from build123d import *

# Parameters (mm, degrees)
SKETCH2_W                          = 128
SKETCH2_H                          = 80
BASE_PLATE_DEPTH                   = 10
PIVOT_PEDESTAL_START               = 10
SKETCH3_R                          = 6
PIVOT_PEDESTAL_DEPTH               = 16
SKETCH4_R                          = 2.7
PIVOT_CLEARANCE_DEPTH              = 26
SKETCH5_R                          = 3.15
LOCATOR_CLEARANCE_DEPTH            = 10
SKETCH6_R                          = 3.15
CUT_EXTRUDE3_DEPTH                 = 10
SKETCH7_R                          = 3.15
SIDE_LOCATOR_CLEARANCE_DEPTH       = 10
LOCATOR_SHOULDER_COUNTERBORE_START = 8
SKETCH8_R                          = 4.1
LOCATOR_SHOULDER_COUNTERBORE_DEPTH = 2
CUT_EXTRUDE6_START                 = 8
SKETCH9_R                          = 4.1
CUT_EXTRUDE6_DEPTH                 = 2
SIDE_SHOULDER_COUNTERBORE_START    = 8
SKETCH10_R                         = 4.1
SIDE_SHOULDER_COUNTERBORE_DEPTH    = 2
SKETCH11_R                         = 3.3
BENCH_MOUNT_M6_CLEARANCE_DEPTH     = 10
SKETCH12_R                         = 3.3
CUT_EXTRUDE9_DEPTH                 = 10
SKETCH13_R                         = 3.3
CUT_EXTRUDE10_DEPTH                = 10
SKETCH14_R                         = 3.3
CUT_EXTRUDE11_DEPTH                = 10


with BuildPart() as part:
    # Sketch2 → Base_plate (new body)
    with BuildSketch(Plane.XY):
        Rectangle(SKETCH2_W, SKETCH2_H)
    extrude(amount=BASE_PLATE_DEPTH)

    # Sketch3 → Pivot_pedestal (add)
    with BuildSketch(Plane.XY.offset(PIVOT_PEDESTAL_START)):
        with Locations(Location((-35, 0, 0), (0, 0, 180))):
            Circle(SKETCH3_R)
    extrude(amount=PIVOT_PEDESTAL_DEPTH)

    # Sketch4 → Pivot_clearance (cut)
    with BuildSketch(Plane.XY):
        with Locations(Location((-35, 0, 0), (0, 0, 180))):
            Circle(SKETCH4_R)
    extrude(amount=PIVOT_CLEARANCE_DEPTH, mode=Mode.SUBTRACT)

    # Sketch5 → Locator_clearance (cut)
    with BuildSketch(Plane.XY):
        with Locations((-10, 15)):
            Circle(SKETCH5_R)
    extrude(amount=LOCATOR_CLEARANCE_DEPTH, mode=Mode.SUBTRACT)

    # Sketch6 → Cut-Extrude3 (cut)
    with BuildSketch(Plane.XY):
        with Locations((10, 15)):
            Circle(SKETCH6_R)
    extrude(amount=CUT_EXTRUDE3_DEPTH, mode=Mode.SUBTRACT)

    # Sketch7 → Side_locator_clearance (cut)
    with BuildSketch(Plane.XY):
        with Locations((-18, -5)):
            Circle(SKETCH7_R)
    extrude(amount=SIDE_LOCATOR_CLEARANCE_DEPTH, mode=Mode.SUBTRACT)

    # Sketch8 → Locator_shoulder_counterbore (cut)
    with BuildSketch(Plane.XY.offset(LOCATOR_SHOULDER_COUNTERBORE_START)):
        with Locations((-10, 15)):
            Circle(SKETCH8_R)
    extrude(amount=LOCATOR_SHOULDER_COUNTERBORE_DEPTH, mode=Mode.SUBTRACT)

    # Sketch9 → Cut-Extrude6 (cut)
    with BuildSketch(Plane.XY.offset(CUT_EXTRUDE6_START)):
        with Locations((10, 15)):
            Circle(SKETCH9_R)
    extrude(amount=CUT_EXTRUDE6_DEPTH, mode=Mode.SUBTRACT)

    # Sketch10 → Side_shoulder_counterbore (cut)
    with BuildSketch(Plane.XY.offset(SIDE_SHOULDER_COUNTERBORE_START)):
        with Locations((-18, -5)):
            Circle(SKETCH10_R)
    extrude(amount=SIDE_SHOULDER_COUNTERBORE_DEPTH, mode=Mode.SUBTRACT)

    # Sketch11 → Bench_mount_M6_clearance (cut)
    with BuildSketch(Plane.XY):
        with Locations((-54, -30)):
            Circle(SKETCH11_R)
    extrude(amount=BENCH_MOUNT_M6_CLEARANCE_DEPTH, mode=Mode.SUBTRACT)

    # Sketch12 → Cut-Extrude9 (cut)
    with BuildSketch(Plane.XY):
        with Locations((-54, 30)):
            Circle(SKETCH12_R)
    extrude(amount=CUT_EXTRUDE9_DEPTH, mode=Mode.SUBTRACT)

    # Sketch13 → Cut-Extrude10 (cut)
    with BuildSketch(Plane.XY):
        with Locations((54, -30)):
            Circle(SKETCH13_R)
    extrude(amount=CUT_EXTRUDE10_DEPTH, mode=Mode.SUBTRACT)

    # Sketch14 → Cut-Extrude11 (cut)
    with BuildSketch(Plane.XY):
        with Locations((54, 30)):
            Circle(SKETCH14_R)
    extrude(amount=CUT_EXTRUDE11_DEPTH, mode=Mode.SUBTRACT)


solid = part.part
CAD build for the part. Positions are in the model's coordinates, mm. A direction names the side the tool comes from. Round coordinates to 2 decimals unless told otherwise and drop trailing zeros. Loops run counter-clockwise (first coordinate to the right, second up) from the corner with the lowest first, then second, coordinate; pieces in that order, holes last.
(1) Cut at A-A (x = -18). Give the cut face in (y, z), plus the area to 3 significant figures.
(2) Cut at B-B (y = 30). Give the cut face in (x, z), plus the area to 3 significant figures.
(3) Cut at D-D (z = 2.75). State how many separate pieces and enclosed holes the cut face has, plus the area to 3 significant figures.
(4) Two-plate mould, pull along Y, no slides. Class faces 1 (the flat face through (-8, 12, 8)), 2 (the flat face through (-1, 40, 5)), 3 (the flat face through (64, -1, 5)), 4 (the flat face through (-1, -40, 5)): +Y half, -Y half, draft (parallel to the pull), parting line (faces both ways), or undercut.
(5) Drop flat-ended pins along their axis: pin 1 (6.5 mm diameter, centred on x = 12, y = 14, fed in from +Z); pin 2 (10.5 mm diameter, centred on x = -10, y = 15, fed in from -Z); pin 3 (1 mm diameter, centred on y = 3.5, z = 11.5, fed in from +X); pin 4 (7.5 mm diameter, centred on x = 10, y = 15, fed in from +Z). Give the stop position or say it passes through.
(6) Cut at C-C (x = 54). Give the cut face in (y, z).
(7) Which spindle directions (+Z, -Z, +X, -X, +Y, -Y) get a long thin tool onto all of the face, cutting with end or side? Do faces 5 (the cylindrical face through (-14.096, 15.18, 8.986)), 6 (the cylindrical face through (-37.575, -0.811, 12.818)). Say none if no direction does.
(8) Wall check: line 1 along Y through (x, z) = (-54, 3); line 2 along Y through (x, z) = (10, 2.25); line 3 along Y through (x, z) = (-10, 8.5). Give the ranges that are in metal, low to high.
Findings below:
1. outline: (-40, 0) - (-8.15, 0) - (-8.15, 8) - (-9.1, 8) - (-9.1, 10) - (-40, 10) - close; (-1.85, 0) - (40, 0) - (40, 10) - (-0.9, 10) - (-0.9, 8) - (-1.85, 8) - close
1. area: 733 mm2
2. outline: (-64, 0) - (-57.3, 0) - (-57.3, 10) - (-64, 10) - close; (-50.7, 0) - (50.7, 0) - (50.7, 10) - (-50.7, 10) - close; (57.3, 0) - (64, 0) - (64, 10) - (57.3, 10) - close
2. area: 1,150 mm2
3. separate pieces: 1
3. enclosed holes: 8
3. area: 9,990 mm2
4. face 1: undercut
4. face 2: +Y half
4. face 3: draft
4. face 4: -Y half
5. pin 1: stops at z = 10
5. pin 2: stops at z = 0
5. pin 3: stops at x = -29.8
5. pin 4: stops at z = 8
6. outline: (-40, 0) - (-33.3, 0) - (-33.3, 10) - (-40, 10) - close; (-26.7, 0) - (26.7, 0) - (26.7, 10) - (-26.7, 10) - close; (33.3, 0) - (40, 0) - (40, 10) - (33.3, 10) - close
7. face 5: +Z
7. face 6: +Z, -Z
8. line 1: y = -40 to -33.3, -26.7 to 26.7, 33.3 to 40
8. line 2: y = -40 to 11.85, 18.15 to 40
8. line 3: y = -40 to 10.9, 19.1 to 40
